Could you check a few things on this model? Use its own coordinates, in mm. Face numbers are marked on the shaded views. A direction names the side the tool comes from. Give positions to 0.01 mm unless a question says otherwise; leave off trailing zeros. Write each loop counter-clockwise with the first axis right and the second up, starting at its lowest first coordinate (ties: lowest second). Pieces come first, ordered by that corner, then holes. Notation, with made-up numbers: M 69.25,89.5 L 126.25,89.5 A14 cw 126.25,94.5 Z; hole C 15,74.25 d11. An arc over 180 degrees is marked long. Use one line per item in the form item = value.
from build123d import *

# Parameters (mm, degrees)
SKETCH_2_R      = 1
EXTRUDE_1_DEPTH = 10
EXTRUDE_2_DEPTH = 6


with BuildPart() as part:
    # 草图1 → 旋转1 (revolve)
    with BuildSketch(Plane(origin=(0, 0, 0), x_dir=(1, 0, 0), z_dir=(0, 1, 0))):
        with BuildLine():
            Line((0, 3), (0, -3))
            ThreePointArc((0, -3), (3, 0), (0, 3))
        make_face()
    revolve(axis=Axis((0, 0, -3), (0, 0, 1)))

    # 草图2 → 凸台-拉伸1 (add)
    with BuildSketch(Plane(origin=(0, 0, 0), x_dir=(1, 0, 0), z_dir=(0, 1, 0))):
        with Locations(Location((0, 0, 0), (0, 0, 90))):
            Circle(SKETCH_2_R)
    extrude(amount=EXTRUDE_1_DEPTH)

    # 草图3 → 凸台-拉伸2 (add)
    with BuildSketch(Plane(origin=(0, 0, 0), x_dir=(1, 0, 0), z_dir=(0, 1, 0))):
        Polygon((2.309401077, 0), (1.154700538, 2), (-1.154700538, 2), (-2.309401077, 0), (-1.154700538, -2), (1.154700538, -2), align=None)
    extrude(amount=EXTRUDE_2_DEPTH)


solid = part.part
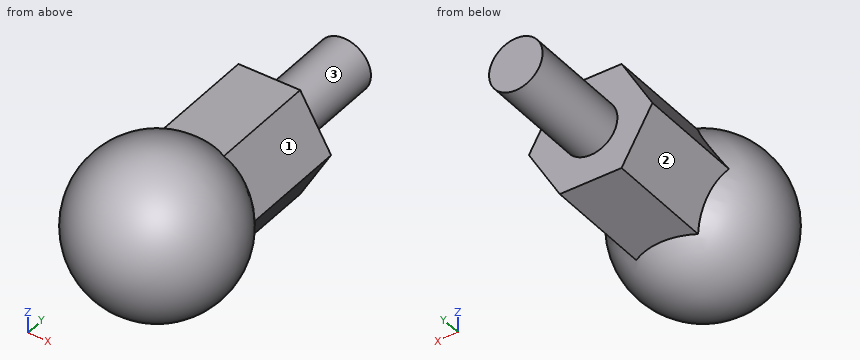
1) I want a section at A-A, the plane x = 0. Please give me the cut outline in (y, z), plus the area to 3 significant figures.
Checked values:
outline = M 2.24,-2 L 6,-2 L 6,-1 L 10,-1 L 10,1 L 6,1 L 6,2 L 2.24,2 A3 ccw long Z
area = 49.2 mm2
2) I want a section at C-C, the plane y = 4.25. Please give me the cut outline in (x, z).
Checked values:
outline = M -2.31,0 L -1.15,-2 L 1.15,-2 L 2.31,0 L 1.15,2 L -1.15,2 Z
3) I want a section at D-D, the plane y = 7.25. Please give me the cut outline in (x, z).
Checked values:
outline = C 0,0 d2
4) If I drill on L1, parallel to Z at x = 0.75, y = 1; L2, parallel to X at y = 3.25, z = 1.5; L3, parallel to X at y = -0.25, z = -2.7, over which ranges is the centre line in solid material (lowest first)?
Checked values:
L1 = -2.73 to 2.73
L2 = -1.44 to 1.44
L3 = -1.28 to 1.28
5) For pin 1 Ø1.2 at (x, y) = (0.5, 4.5) entering from -Z; pin 2 Ø1.8 at (x, y) = (-0.5, 5) entering from +Z; pin 3 Ø1 at (y, z) = (-1, 0) entering from -X, each with a flat end and sliding along its axis, tell me the tip position at first contact or that it passes through.
Checked values:
pin_1 = -2
pin_2 = 2
pin_3 = -2.96
6) For the marked faces 1, 2 and 3, which set-ups out of +Z, -Z, +X, -X, +Y, -Y let a thin tool reach every point of the face, with its end or its side?
Checked values:
face_1 = +Z, +X, +Y
face_2 = -Z, -X, +Y
face_3 = +Y
7) I want a section at B-B, the plane z = -0.3. Please give me the cut outline in (x, y), plus the area to 3 significant figures.
Checked values:
outline = M -2.14,2.08 A2.98 ccw long 2.14,2.08 L 2.14,6 L 0.95,6 L 0.95,10 L -0.95,10 L -0.95,6 L -2.14,6 Z
area = 49.7 mm2
